from build123d import *

# Parameters (mm, degrees)
SKETCH_2_R      = 1.7
SKETCH_2_R_2    = 2.6
SKETCH_2_R_3    = 11.2
SKETCH_2_R_4    = 3.655
SKETCH_2_R_5    = 3
EXTRUDE_1_DEPTH = 6
CHAMFER_1_SIZE  = 1
CHAMFER_2_SIZE  = 0.5
FILLET_1_R      = 0.5


with BuildPart() as part:
    # Эскиз2 → Бобышка-Вытянуть1 (new body)
    with BuildSketch(Plane(origin=(0, 0, 0), x_dir=(0, 0, -1), z_dir=(1, 0, 0))):
        with BuildLine():
            Line((-28.783294421, 72.542236653), (28.783294421, 72.542236653))
            ThreePointArc((28.783294421, 72.542236653), (36.714702999, 69.256939651), (40, 61.325531074))
            Line((40, 61.325531074), (40, -30.391408151))
            ThreePointArc((40, -30.391408151), (39.238795325, -34.218242474), (37.071067812, -37.462475962))
            Line((37.071067812, -37.462475962), (2.828427125, -71.70511665))
            ThreePointArc((2.828427125, -71.70511665), (0, -72.876689525), (-2.828427125, -71.70511665))
            Line((-2.828427125, -71.70511665), (-37.071067812, -37.462475962))
            ThreePointArc((-37.071067812, -37.462475962), (-39.238795325, -34.218242474), (-40, -30.391408151))
            Line((-40, -30.391408151), (-40, 61.325531074))
            ThreePointArc((-40, 61.325531074), (-36.714702999, 69.256939651), (-28.783294421, 72.542236653))
        make_face()
        with Locations((-21.913410217, -46.3871)):
            Circle(SKETCH_2_R, mode=Mode.SUBTRACT)
        with Locations((17.25, -19.8871)):
            Circle(SKETCH_2_R_2, mode=Mode.SUBTRACT)
        with Locations((-17.25, -19.8871)):
            Circle(SKETCH_2_R_2, mode=Mode.SUBTRACT)
        with Locations((0.0069, -46.3871)):
            Circle(SKETCH_2_R_3, mode=Mode.SUBTRACT)
        with Locations((-25, 37.1129)):
            Circle(SKETCH_2_R_4, mode=Mode.SUBTRACT)
        with Locations((-20, 63.3206)):
            Circle(SKETCH_2_R_5, mode=Mode.SUBTRACT)
        with Locations((0, 63.3206)):
            Circle(SKETCH_2_R_5, mode=Mode.SUBTRACT)
        with Locations((0, 43.3206)):
            Circle(SKETCH_2_R_5, mode=Mode.SUBTRACT)
        with Locations((20, 63.3206)):
            Circle(SKETCH_2_R_5, mode=Mode.SUBTRACT)
        with Locations((25, 37.1129)):
            Circle(SKETCH_2_R_4, mode=Mode.SUBTRACT)
        with Locations((0.0069, -24.466789783)):
            Circle(SKETCH_2_R, mode=Mode.SUBTRACT)
        with Locations((21.927210217, -46.3871)):
            Circle(SKETCH_2_R, mode=Mode.SUBTRACT)
        with Locations((0.0069, -68.307410217)):
            Circle(SKETCH_2_R, mode=Mode.SUBTRACT)
    extrude(amount=EXTRUDE_1_DEPTH)

    # Фаска1
    chamfer_1_edges = [part.edges().sort_by_distance(p)[0] for p in [
        (6, -19.8871, -14.65),
        (6, -19.8871, 19.85),
        (6, 63.3206, 23),
        (6, 63.3206, 3),
        (6, 43.3206, 3),
        (6, 63.3206, -17),
    ]]
    chamfer(chamfer_1_edges, length=CHAMFER_1_SIZE)

    # Фаска2
    chamfer_2_edges = [part.edges().sort_by_distance(p)[0] for p in [
        (6, -24.466789783, 1.6931),
        (6, -46.3871, 23.613410217),
        (6, -46.3871, -20.227210217),
        (6, -68.307410217, 1.6931),
    ]]
    chamfer(chamfer_2_edges, length=CHAMFER_2_SIZE)

    # Скругление1
    fillet_1_edges = [part.edges().sort_by_distance(p)[0] for p in [
        (6, -34.218242474, -39.238795325),
        (6, 15.467061462, -40),
        (6, 69.256939651, -36.714702999),
        (6, 72.542236653, 0),
        (6, 69.256939651, 36.714702999),
        (6, 15.467061462, 40),
        (6, -34.218242474, 39.238795325),
        (6, -54.583796306, 19.949747468),
        (6, -72.876689525, 0),
        (6, -46.3871, 11.1931),
        (6, -54.583796306, -19.949747468),
    ]]
    fillet(fillet_1_edges, radius=FILLET_1_R)


solid = part.part
Here's how the part is built. I have some questions about the finished solid (model axes, mm). Give positions to 0.01 mm unless a question says otherwise; leave off trailing zeros. One line per item, written item: value. Start each with the question number.
1. I need wall thicknesses on probe 1 along Y at (x, z) = (5.75, 22); probe 2 along Y at (x, z) = (2, 17.5); probe 3 along Y at (x, z) = (4.75, -19). Which ranges of each line are inside material? Lowest first, please. Write a range as from..to.
2. We'd pull the mould along Y, two halves only. Please class faces 1 (the face through (3, 15, 40)), 2 (the face through (2.958, 39.583, 27.694)), 3 (the face through (2.712, -72.876, -0.044)), 4 (the face through (2.465, 63.453, 22.997)): released by +Y, released by -Y, zero draft, split by the parting line, or undercut.
3. Imagine slicing it at A-A, the plane x = 2.5. Count the separate pieces of the cut face and the enclosed holes in it, plus the area to 3 significant figures.
4. Will this pin go through, and if not, where does the flat tip stop? pin 1 Ø7 at (y, z) = (-19.89, 17.25) entering from +X.
Values follow:
1. probe 1: y = -52.44..-48.34, -44.44..35.03, 39.2..60.15, 66.49..72.48
1. probe 2: y = -57.03..-22.48, -17.3..61.66, 64.98..72.54
1. probe 3: y = -55.53..-21.81, -17.96..60.49, 66.15..72.54
2. face 1: zero draft
2. face 2: undercut
2. face 3: released by -Y
2. face 4: undercut
3. separate pieces: 1
3. enclosed holes: 13
3. area: 9,430 mm2
4. pin 1: stops at x = 5.9
